The drawing under review shows one solid part. Ordinate dimensions are in mm from its lowest x, y, z. A direction names the side the tool comes from. Give positions to 0.01 mm unless a question says otherwise; leave off trailing zeros. Order: outer loops, then holes, each group sorted by start corner. A loop starts at its lowest first (then second) coordinate and runs counter-clockwise, first axis right, second up. Notation, with made-up numbers: M -31,73 L -1,73 A20 cw -1,106 Z; hole C -32,-24.5 d5. An arc over 180 degrees is marked long. Put each result on its own line as item: value. Start each with the question number.
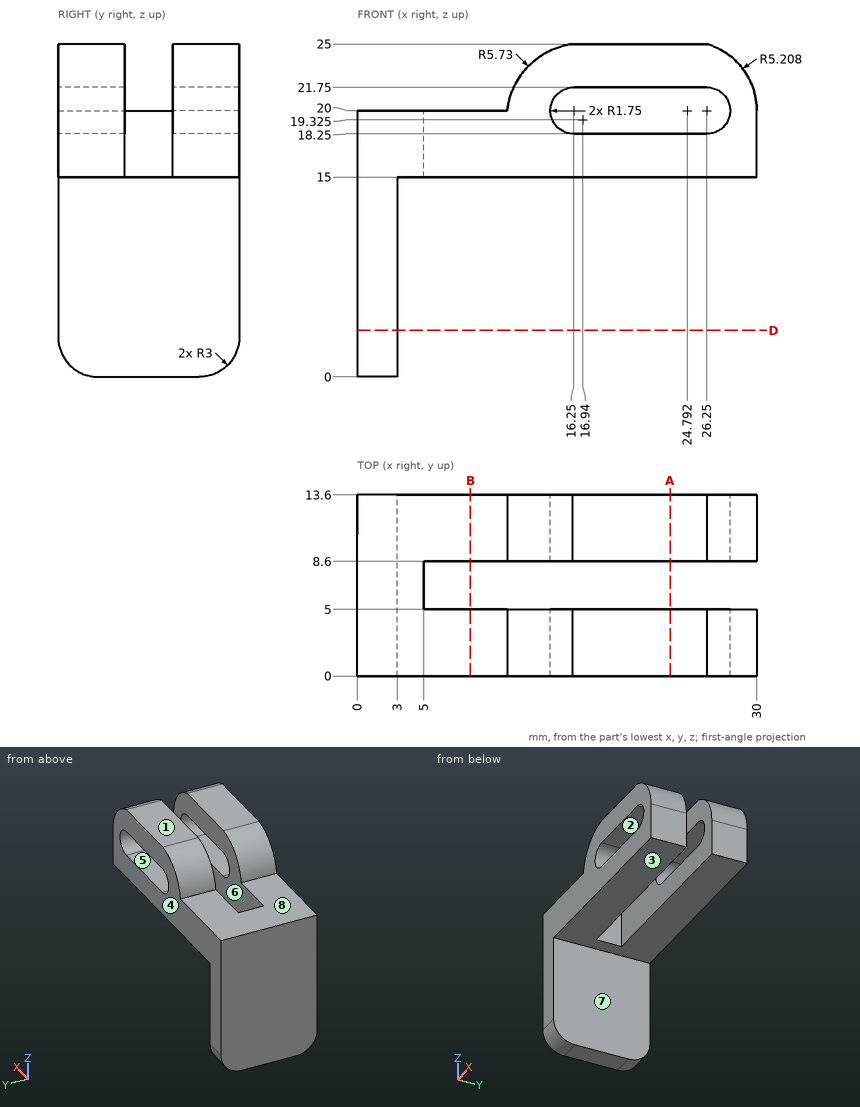
1. To check wall thickness, follow probe 1 along Z at (x, y) = (18.25, 2.25); probe 2 along Y at (x, z) = (6.5, 18.5); probe 3 along X at (y, z) = (10.5, 13.5). State the ranges of each line that lie inside material, in increasing order.
2. Consider section A-A on x = 23.5. Give the boundary of the cut face in (y, z).
3. Insertion check: pin 1 (6 mm diameter, centred on x = 11.5, y = 7, fed in from -Z); pin 2 (1.5 mm diameter, centred on y = 4, z = 8, fed in from +X); pin 3 (5.5 mm diameter, centred on x = 5.5, y = 4, fed in from +Z). Each pin has a flat end and moves straight along its axis. Give the tip position at first contact, or say it passes through.
4. Consider section B-B on x = 8.5. Give the boundary of the cut face in (y, z), then the cut area to 3 significant figures.
5. The part is to be moulded in two halves that separate along Z. For the marked faces 1, 2, 3 and 4, say which applies: +Z half, -Z half, draft (parallel to the pull), parting line (faces both ways), or undercut.
6. Machinability: for the marked faces 5, 6, 7 and 8, which of the approach directions +Z, -Z, +X, -X, +Y, -Y give a long, thin tool a straight path to every point of the face, cutting with its end or side? Answer none if there is none.
7. Consider section D-D on z = 3.5. Give the boundary of the cut face in (x, y), then the cut area to 3 significant figures.
Returned:
1. probe 1: z = 15 to 18.25, 21.75 to 25
1. probe 2: y = 0 to 5, 8.6 to 13.6
1. probe 3: x = 0 to 3
2. outline: M 0,15 L 5,15 L 5,18.25 L 0,18.25 Z; M 0,21.75 L 5,21.75 L 5,25 L 0,25 Z; M 8.6,15 L 13.6,15 L 13.6,18.25 L 8.6,18.25 Z; M 8.6,21.75 L 13.6,21.75 L 13.6,25 L 8.6,25 Z
3. pin 1: stops at z = 15
3. pin 2: stops at x = 3
3. pin 3: stops at z = 20
4. outline: M 0,15 L 5,15 L 5,20 L 0,20 Z; M 8.6,15 L 13.6,15 L 13.6,20 L 8.6,20 Z
4. area: 50.0 mm2
5. face 1: +Z half
5. face 2: undercut
5. face 3: -Z half
5. face 4: draft
6. face 5: +Y, -Y
6. face 6: +Z, -Z, +X
6. face 7: -Z, +X, +Y, -Y
6. face 8: +Z, -X, +Y, -Y
7. outline: M 0,0 L 3,0 L 3,13.6 L 0,13.6 Z
7. area: 40.8 mm2
